The listing builds one solid part. Answer for the finished solid, in the listing's coordinates (mm). A direction names the side the tool comes from. Give positions to 0.01 mm unless a question says otherwise; leave off trailing zeros. Order: outer loops, then holes, each group sorted by start corner. A loop starts at its lowest first (then second) coordinate and runs counter-clockwise, first axis right, second up. Notation, with made-up numbers: (40.5, 53) - (78.5, 53) arc R18 ccw to (78.5, 79) - close; hole circle Ø3 at (19, 58). An arc over 180 degrees is marked (long way). Write each question's results on one line, items separated by ' | '. Start each with the question number.
1. Section B-B (x = -8.25) is taken. Give the vertices of the cut face in (y, z), and give its area (3 significant figures).
2. Which of the six approach directions +Z, -Z, +X, -X, +Y, -Y give full straight-line access (tool end or side, diameter ignored) to faces 4 (the face through (-8, 39.5, -55)), 5 (the face through (-8, -39.5, -55)), 6 (the face through (-3.48, 29.16, 14.73)), 7 (the face through (-8, 39.5, 55))?
3. Section A-A (y = 0) is taken. Give the vertices of the cut face in (x, z).
4. Section C-C (z = -54.5) is taken. Give the vertices of the cut face in (x, y), and give its area (3 significant figures).
5. Determine the mould class of faces 1 (the face through (-7, -38, 51.5)), 2 (the face through (-2, 30.8, -19.3)), 3 (the face through (-3, -27.5, -42)) for opening direction Y: released by +Y, released by -Y, zero draft, split by the parting line, or undercut.
6. Section D-D (y = -12) is taken. Give the vertices of the cut face in (x, z).
7. Find the intervals of material crossed by L1, parallel to Y at x = -1.05, z = 35; L2, parallel to Z at x = -2.5, y = -36; L3, parallel to Y at x = -3.65, z = -35, in increasing order.
8. Flat-ended cylindrical pins translate along their axes: pin 1 (5 mm diameter, centred on y = 17.5, z = 3.5, fed in from -X); pin 2 (3.5 mm diameter, centred on x = -9.5, z = -56, fed in from +Y); pin 3 (1.5 mm diameter, centred on x = -2, z = -64.5, fed in from -Y); pin 4 (2 mm diameter, centred on y = -30.31, z = 17.5, fed in from -X) (1 decimal). Find the tip coordinate at first contact, or state that the pin passes through.
Autodesk Inventor part; units mm, degrees
ref_plane "Work Plane1" through (-2, 0, 0) normal (1, 0, 0) x (0, 0, -1)
ref_plane "YZ Plane" through (0, 0, 0) normal (1, 0, 0) x (0, 1, 0)
ref_plane "XZ Plane" through (0, 0, 0) normal (0, 1, 0) x (-1, 0, 0)
sketch "Sketch1" plane through (0, 0, 0) normal (0, 0, 1) x (1, 0, 0)
  line L0 (0, 0) -> (0, 44)
  line L1 (-5, 0) -> (0, 0)
  line L2 (0, 44) -> (-1, 44)
  line L3 (-1, 44) -> (-5, 40)
  line L4 (-5, 40) -> (-5, 0)
  dimension "d0" = 44
  dimension "d3" = 1
  dimension "d19" = 5
  dimension "d20" = 45
revolve "Revolution1" add sketch "Sketch1" angle 360 about axis through (-5, 0, 0) along (1, 0, 0)
sketch "Sketch2" plane through (0, 0, 0) normal (1, 0, 0) x (0, 0, -1)
  line L0 (0, 0) -> (35, 0) construction
  circle A0 centre (35, 0) radius 1.65
  dimension "d7" = 3.3
  dimension "d8" = 35
extrude "Extrusion1" cut sketch "Sketch2" against normal through all
ref_plane "Work Plane1" through (-2, 0, 0) normal (1, 0, 0) x (0, 0, -1)
sketch "Sketch3" plane through (-2, 0, 0) normal (1, 0, 0) x (0, 0, -1)
  circle A0 centre (35, 0) radius 3
  circle A1 centre (35, 0) radius 1.65
  point P0 (0, 0)
  dimension "d12" = 6
extrude "Extrusion2" cut sketch "Sketch3" against normal through all contours A0 | A1
pattern_circular "Circular Pattern1" count 6 over 360 about axis through (-0.5, 0, 0) along (1, 0, 0) of "Extrusion2", "Extrusion1"
sketch "Sketch4" plane through (-5, 0, 0) normal (-1, 0, 0) x (0, 0, 1)
  line L0 (73.5, 27.5) -> (-73.5, 27.5)
  line L1 (-73.5, 27.5) -> (-73.5, -27.5)
  line L2 (-73.5, -27.5) -> (73.5, -27.5)
  line L3 (73.5, -27.5) -> (73.5, 27.5)
  line L4 (73.5, 27.5) -> (-73.5, -27.5) construction
  line L5 (-73.5, 27.5) -> (73.5, -27.5) construction
  line L6 (58.5, -27.5) -> (51.5, -27.5)
  line L7 (51.5, -27.5) -> (51.5, -37.5)
  line L8 (51.5, -37.5) -> (58.5, -37.5)
  line L9 (58.5, -37.5) -> (58.5, -27.5)
  line L10 (-51.5, -27.5) -> (-58.5, -27.5)
  line L11 (-58.5, -27.5) -> (-58.5, -37.5)
  line L12 (-58.5, -37.5) -> (-51.5, -37.5)
  line L13 (-51.5, -37.5) -> (-51.5, -27.5)
  line L14 (-51.5, 27.5) -> (-58.5, 27.5)
  line L15 (-58.5, 27.5) -> (-58.5, 37.5)
  line L16 (-58.5, 37.5) -> (-51.5, 37.5)
  line L17 (-51.5, 37.5) -> (-51.5, 27.5)
  line L18 (58.5, 27.5) -> (51.5, 27.5)
  line L19 (51.5, 27.5) -> (51.5, 37.5)
  line L20 (51.5, 37.5) -> (58.5, 37.5)
  line L21 (58.5, 37.5) -> (58.5, 27.5)
  circle A0 centre (0, 0) radius 40
  point P0 (-29.0474, -27.5)
  point P1 (-29.0474, 27.5)
  point P2 (29.0474, 27.5)
  point P3 (29.0474, -27.5)
  dimension "d21" = 147
  dimension "d22" = 55
  dimension "d23" = 15
  dimension "d24" = 7
  dimension "d26" = 15
  dimension "d29" = 75
extrude "Extrusion3" add sketch "Sketch4" against normal up to surface (5 mm away) contours L3 L2 A0 L0 | L0 L19 L20 L21 | L9 L8 L7 L2 | A0 L2 L1 L0 | L0 L15 L16 L17 | L13 L12 L11 L2
sketch "Sketch5" plane through (-5, 27.5, -58.5) normal (0, 0, -1) x (-1, 0, 0)
  line L0 (-5, -65) -> (10.6, -65)
  line L1 (12.6, -65) -> (12.6, -67)
  line L2 (12.6, -67) -> (-5, -67)
  line L3 (-5, -67) -> (-5, -65)
  line L4 (-5, 10) -> (10.6, 10)
  line L5 (12.6, 10) -> (12.6, 12)
  line L6 (12.6, 12) -> (-5, 12)
  line L7 (-5, 12) -> (-5, 10)
  line L8 (10.6, 10) -> (10.6, 8.5)
  line L9 (10.6, 8.5) -> (12.6, 8.5)
  line L10 (12.6, 8.5) -> (12.6, 10)
  line L11 (10.6, -65) -> (10.6, -63.5)
  line L12 (10.6, -63.5) -> (12.6, -63.5)
  line L13 (12.6, -63.5) -> (12.6, -65)
  line L14 (0, 10) -> (0, 0)
  point P0 (-5, -27.5)
  dimension "d30" = 2
  dimension "d31" = 10.6
  dimension "d32" = 2
  dimension "d33" = 1.5
extrude "Extrusion4" add sketch "Sketch5" against normal up to surface (7 mm away)
sketch "Sketch6" plane through (-5, -37.5, 51.5) normal (0, 0, -1) x (-1, 0, 0)
  line L0 (-5, 77) -> (-5, 65)
  line L1 (0, 65) -> (-5, 65)
  line L2 (0, 75) -> (0, 65)
  line L3 (0, 75) -> (10.6, 75)
  line L4 (10.6, 75) -> (10.6, 73.5)
  line L5 (10.6, 73.5) -> (12.6, 73.5)
  line L6 (12.6, 73.5) -> (12.6, 77)
  line L7 (12.6, 77) -> (-5, 77)
  line L8 (-5, 10) -> (-5, -2)
  line L9 (-5, -2) -> (12.6, -2)
  line L10 (12.6, -2) -> (12.6, 1.5)
  line L11 (12.6, 1.5) -> (10.6, 1.5)
  line L12 (10.6, 1.5) -> (10.6, 0)
  line L13 (10.6, 0) -> (0, 0)
  line L14 (0, 10) -> (0, 0)
  line L15 (0, 10) -> (-5, 10)
  point P0 (-5, 37.5)
extrude "Extrusion5" add sketch "Sketch6" against normal up to surface (7 mm away)
fillet "Fillet1" radius 5 4 edges at (-2.5, -27.5, -73.5) (-2.5, 27.5, -73.5) (-2.5, -27.5, 73.5) (-2.5, 27.5, 73.5)
fillet "Fillet2" radius 2 4 edges at (-17.6, 39.5, 55) (-17.6, 39.5, -55) (-17.6, -39.5, 55) (-17.6, -39.5, -55)
fillet "Fillet3" radius 2 8 edges at (-2.5, 27.5, -58.5) (-2.5, 27.5, 51.5) (-2.5, -27.5, 51.5) (-2.5, -27.5, -58.5) (-2.5, -27.5, -51.5) (-2.5, -27.5, 58.5) (-2.5, 27.5, 58.5) (-2.5, 27.5, -51.5)
properties part number "PhoneHOldER"
Reported:
1) outline: (-39.5, -58.5) - (-37.5, -58.5) - (-37.5, -51.5) - (-39.5, -51.5) - close; (-39.5, 51.5) - (-37.5, 51.5) - (-37.5, 58.5) - (-39.5, 58.5) - close; (37.5, -58.5) - (39.5, -58.5) - (39.5, -51.5) - (37.5, -51.5) - close; (37.5, 51.5) - (39.5, 51.5) - (39.5, 58.5) - (37.5, 58.5) - close | area: 56.0 mm²
2) face 4: -Z, +X, -X, +Y | face 5: -Z, +X, -X, -Y | face 6: -X | face 7: +Z, +X, -X, +Y
3) outline: (-5, -73.5) - (0, -73.5) - (0, -36.65) - (-2, -36.65) - (-2, -38) - (-5, -38) - close; (-5, -32) - (-2, -32) - (-2, -33.35) - (0, -33.35) - (0, 33.35) - (-2, 33.35) - (-2, 32) - (-5, 32) - close; (-5, 38) - (-2, 38) - (-2, 36.65) - (0, 36.65) - (0, 73.5) - (-5, 73.5) - close
4) outline: (-17.6, -37.5) arc R2 ccw to (-15.6, -39.5) - (0, -39.5) - (0, 39.5) - (-15.6, 39.5) arc R2 ccw to (-17.6, 37.5) - (-17.6, 36) - (-15.6, 36) - (-15.6, 37.5) - (-5, 37.5) - (-5, -37.5) - (-15.6, -37.5) - (-15.6, -36) - (-17.6, -36) - close | area: 450 mm²
5) face 1: zero draft | face 2: undercut | face 3: released by -Y
6) outline: (-5, -73.5) - (0, -73.5) - (0, 73.5) - (-5, 73.5) - close
7) L1: -27.5 to -1.65, 1.65 to 27.5 | L2: -58.5 to -51.5, -22.59 to 22.59, 51.5 to 58.5 | L3: -27.5 to -3, 3 to 27.5
8) pin 1: x = -5 | pin 2: y = 39.5 | pin 3: y = -27.5 | pin 4: through
